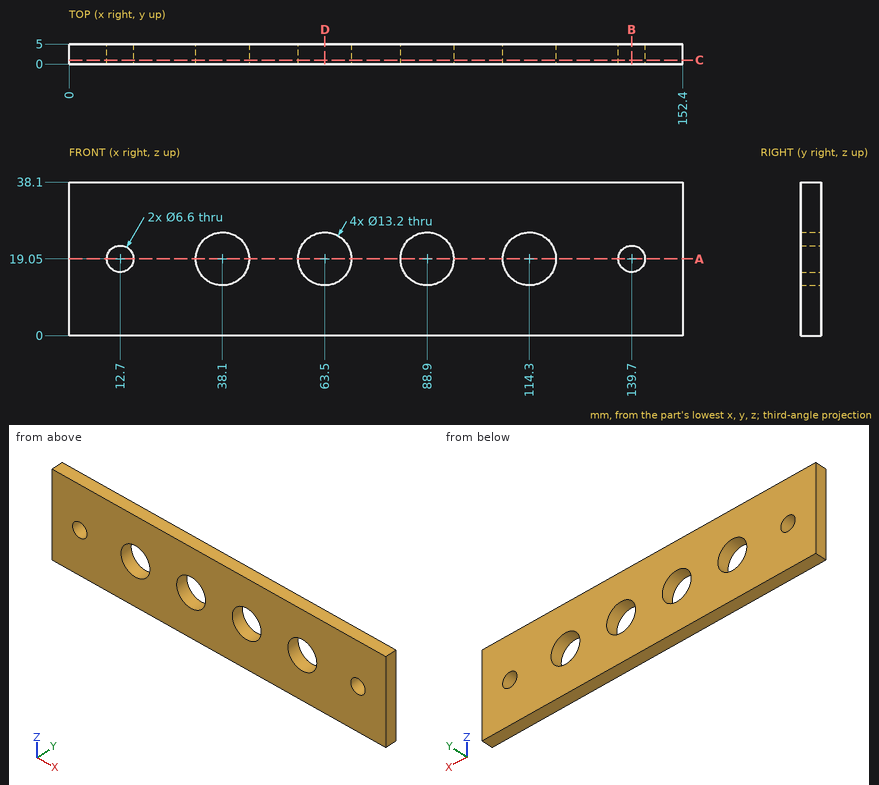
Verification items for this drawing (mm, ordinates from the low corner). Give positions to 0.01 mm unless a question says otherwise; leave off trailing zeros. Write each loop counter-clockwise with the first axis right and the second up, starting at its lowest first coordinate (ties: lowest second). Pieces come first, ordered by that corner, then holes. Notation, with made-up numbers: (43, 62.25) - (101, 62.25) arc R19 ccw to (101, 89.25) - close; hole circle Ø1 at (-6, -11). An arc over 180 degrees is marked (long way). Answer as CSV lines item,"result". Start each with the question number.
1. Thickness scan on line 1 (Z direction, x = 12.7, y = 1.5); line 2 (Z direction, x = 114.3, y = 2.7). Record the ranges inside material, lowest first.
2. Sectioned sample at D-D (x = 63.5). Record the boundary of the cut face in (y, z), then the cut area to 4 significant figures.
3. Sectioned sample at A-A (z = 19.05). Record the boundary of the cut face in (x, y).
4. Depth check by flat-ended pin: pin 1 (10.5 mm diameter, centred on x = 63.5, z = 19.05, fed in from +Y). Enter the tip coordinate at first touch or a pass-through.
5. Sectioned sample at B-B (x = 139.7). Record the boundary of the cut face in (y, z), then the cut area to 4 significant figures.
6. Sectioned sample at C-C (y = 1). Record the boundary of the cut face in (x, z).
Derived:
1,line 1,"0 to 15.75, 22.35 to 38.1"
1,line 2,"0 to 12.45, 25.65 to 38.1"
2,outline,"(0, 0) - (5, 0) - (5, 12.45) - (0, 12.45) - close; (0, 25.65) - (5, 25.65) - (5, 38.1) - (0, 38.1) - close"
2,area,"124.5 mm²"
3,outline,"(0, 0) - (9.4, 0) - (9.4, 5) - (0, 5) - close; (16, 0) - (31.5, 0) - (31.5, 5) - (16, 5) - close; (44.7, 0) - (56.9, 0) - (56.9, 5) - (44.7, 5) - close; (70.1, 0) - (82.3, 0) - (82.3, 5) - (70.1, 5) - close; (95.5, 0) - (107.7, 0) - (107.7, 5) - (95.5, 5) - close; (120.9, 0) - (136.4, 0) - (136.4, 5) - (120.9, 5) - close; (143, 0) - (152.4, 0) - (152.4, 5) - (143, 5) - close"
4,pin 1,"through"
5,outline,"(0, 0) - (5, 0) - (5, 15.75) - (0, 15.75) - close; (0, 22.35) - (5, 22.35) - (5, 38.1) - (0, 38.1) - close"
5,area,"157.5 mm²"
6,outline,"(0, 0) - (152.4, 0) - (152.4, 38.1) - (0, 38.1) - close; hole circle Ø6.6 at (12.7, 19.05); hole circle Ø13.2 at (38.1, 19.05); hole circle Ø13.2 at (63.5, 19.05); hole circle Ø13.2 at (88.9, 19.05); hole circle Ø13.2 at (114.3, 19.05); hole circle Ø6.6 at (139.7, 19.05)"
